Autodesk Inventor part; units mm, degrees
ref_plane "YZ Plane" through (0, 0, 0) normal (1, 0, 0) x (0, 1, 0)
ref_plane "XZ Plane" through (0, 0, 0) normal (0, 1, 0) x (-1, 0, 0)
ref_plane "XY Plane" through (0, 0, 0) normal (0, 0, 1) x (1, 0, 0)
sketch "Sketch1" plane through (0, 0, 0) normal (1, 0, 0) x (0, 1, 0)
  line L0 (-39.3892, -105) -> (-110, -20.8494)
  line L1 (-110, -20.8494) -> (-110, 0)
  line L2 (-110, 0) -> (0, 0)
  line L3 (0, 0) -> (0, -105)
  line L4 (0, -105) -> (-39.3892, -105)
  line L5 (-110, -20.8494) -> (-119.38, 0) construction
  line L6 (-119.38, 0) -> (-110, 0) construction
  line L7 (-50.8, -25.4) -> (0, -25.4) construction
  line L8 (0, -25.4) -> (0, 0) construction
  line L9 (0, 0) -> (-50.8, 0) construction
  line L10 (-50.8, 0) -> (-50.8, -25.4) construction
  line L11 (-50.8, -25.4) -> (0, 0) construction
  line L12 (0, -25.4) -> (-50.8, 0) construction
  circle A0 centre (-12.7, -12.7) radius 3
  circle A1 centre (-38.1, -12.7) radius 3
  circle A2 centre (-102.5, -49) radius 14.2875
  circle A3 centre (-25.4, -75) radius 14.2875
  circle A4 centre (-102.5, -49) radius 20
  circle A5 centre (-25.4, -75) radius 30
  line L13 (-50.8, -90.9637) -> (-50.8, -59.0363)
  line L14 (-102.5, -49) -> (-25.4, -75) construction
  point P0 (-25.4, -12.7)
  point P1 (-25.4, -25.4)
  point P2 (-103.1519, -29.0106)
  point P3 (-82.9275, -53.1131)
  point P4 (-50.8, -75)
  point P5 (-48.3813, -94.2836)
  point P6 (0, -90.9637)
  dimension "d0" = 50
  dimension "d1" = 119.38
  dimension "d2" = 50.8
  dimension "d3" = 25.4
  dimension "d4" = 25.4
  dimension "d5" = 12.7
  dimension "d6" = 6
  dimension "d7" = 6
  dimension "d8" = 28.575
  dimension "d9" = 102.5
  dimension "d10" = 49
  dimension "d13" = 110
  dimension "d16" = 60
  dimension "d17" = 25.4
  dimension "d18" = 25.4
  dimension "d20" = 40
  dimension "d44" = 81.3659
extrude "Plate1" add sketch "Sketch1" along normal blind 3.175 contours L0 A4 L1 L2 L3 A5 | A5 L13 L3 | A4 L0 A2 | L0 A2 A4 | A5 L13
fillet "Corner Round1" radius 15 4 edges at (1.5875, -82.9275, -53.1131) (1.5875, -103.1519, -29.0106) (1.5875, -110, -20.8494) (1.5875, -110, 0)
fillet "Corner Round1" radius 6 1 edges at (1.5875, 0, -90.9637)
sketch "Sketch2" plane through (0, 0, 0) normal (-1, 0, 0) x (0, 0, 1)
  circle A0 centre (-31.4501, -106.5) radius 4.5847
  circle A1 centre (-49, -102.5) radius 14.2875
  point P0 (0, 0)
  dimension "d21" = 9.1694
  dimension "d22" = 18
  dimension "d23" = 4
hole "Hole1" at (0, -106.5, -31.4501) direction (1, 0, 0) diameter 3.683 end through all
sketch "Sketch3" plane through (3.175, 0, 0) normal (1, 0, 0) x (0, 0, -1)
  circle A0 centre (75, -25.4) radius 14.2875
  circle A1 centre (75, -25.4) radius 25.4
  line L0 (49.6, -25.4) -> (100.4, -25.4)
  line L1 (92.9605, -7.4395) -> (57.0395, -7.4395)
  line L2 (75, -25.4) -> (57.0395, -7.4395)
  line L3 (92.9605, -43.3605) -> (57.0395, -43.3605)
  line L4 (75, -25.4) -> (92.9605, -43.3605)
  line L5 (25.4, -50.8) -> (0, -50.8)
  line L6 (0, -50.8) -> (0, 0)
  line L7 (0, 0) -> (25.4, 0)
  line L8 (25.4, 0) -> (25.4, -50.8)
  line L9 (25.4, -50.8) -> (0, 0) construction
  line L10 (0, -50.8) -> (25.4, 0) construction
  point P0 (12.7, -25.4)
  dimension "d31" = 50.8
  dimension "d32" = 45
  dimension "d40" = 25.4
  dimension "d41" = 50.8
hole "Hole2" at (3.175, -7.4395, -57.0395) at (3.175, -25.4, -49.6) at (3.175, -43.3605, -57.0395) at (3.175, -43.3605, -92.9605) at (3.175, -25.4, -100.4) at (3.175, -7.4395, -92.9605) direction (-1, 0, 0) diameter 5.105 end through all
equation "\"d7\" = d6"
equation "\"d29\" = Thickness"
equation "\"d14\" = Thickness"
equation "\"BendRadius\" = Thickness"
equation "\"BendReliefWidth\" = Thickness"
equation "\"BendReliefDepth\" = 0.5 * Thickness"
equation "\"CornerReliefSize\" = 4 * Thickness"
equation "\"MinimumRemnant\" = 2 * Thickness"
equation "\"TransitionRadius\" = BendRadius"
equation "\"JacobiRadiusSize\" = BendRadius"
equation "\"GapSize\" = Thickness"
properties part number "INSIDE_INTAKE_PLATE" material "Aluminum, 6061-T6"
Part model, mm, in its own coordinate system. A direction names the side the tool comes from. Round coordinates to 2 decimals unless told otherwise and drop trailing zeros. Write each loop counter-clockwise with the first axis right and the second up, starting at its lowest first coordinate (ties: lowest second). Pieces come first, ordered by that corner, then holes. Notation, with made-up numbers: (27, 19.25) -> (58, 19.25) arc R24 ccw to (58, 31.25) -> close; hole circle Ø2 at (59, -6). An arc over 180 degrees is marked (long way). Return JSON: item names as keys, results as strings. Group by question number.
Q1. Saw through at B-B on z = -49. Write the cut outline in (x, y) (1 decimal).
Q2. Probe L1, parallel to Z at x = 1.75, y = -25.4; L2, parallel to Y at x = 2.4, z = -49.6; L3, parallel to Y at x = 2.3, z = -12. List the from-to ranges inside material, lowest first. Write a range as [from, to].
Q3. Saw through at D-D on y = -102.5. Write the cut outline in (x, z) (1 decimal).
Q4. Pin check, flat tip, straight feed: pin 1 (1 mm diameter, centred on x = 1, z = -16.5, fed in from -Y). Stop position of the tip, or through.
Q5. Mould opens along Z. For faces 1 (the flat face through (2, -48, 0)), 2 (the cylindrical face through (1.565, -27.26, -89.166)), 3 (the flat face through (3.175, -48, -40)) say: pulls with the +Z half, pulls with the -Z half, needs draft (parallel to the pull), parting line crosses it, or undercut.
Q6. Saw through at C-C on x = 1.4. State how many separate pieces and enclosed holes the cut face has, plus the area to 3 significant figures.
Q7. Saw through at A-A on y = -25.4. Write the cut outline in (x, z) (1 decimal).
Q8. Which spindle directions (+Z, -Z, +X, -X, +Y, -Y) get a long thin tool onto all of the face, cutting with end or side? Do faces 4 (the cylindrical face through (1.61, -104.702, -31.849)), 5 (the flat face through (2, -110, -18)). Say none if no direction does.
Answer:
{
 "1": {"outline": "(0, -122.5) -> (3.2, -122.5) -> (3.2, -116.8) -> (0, -116.8) -> close; (0, -88.2) -> (3.2, -88.2) -> (3.2, -27.9) -> (0, -27.9) -> close; (0, -22.9) -> (3.2, -22.9) -> (3.2, 0) -> (0, 0) -> close"},
 "2": {"L1": "[-105, -102.95], [-97.85, -89.29], [-60.71, -52.15], [-47.05, 0]", "L2": "[-122.49, -116.77], [-88.23, -27.95], [-22.85, 0]", "L3": "[-109.7, -41.02], [-35.18, -15.62], [-9.78, 0]"},
 "3": {"outline": "(0, -69) -> (3.2, -69) -> (3.2, -63.3) -> (0, -63.3) -> close; (0, -34.7) -> (3.2, -34.7) -> (3.2, -2) -> (0, -2) -> close"},
 "4": {"pin 1": "y = -110"},
 "5": {"face 1": "pulls with the +Z half", "face 2": "undercut", "face 3": "needs draft"},
 "6": {"separate pieces": "1", "enclosed holes": "11", "area": "8,120 mm2"},
 "7": {"outline": "(0, -105) -> (3.2, -105) -> (3.2, -103) -> (0, -103) -> close; (0, -97.8) -> (3.2, -97.8) -> (3.2, -89.3) -> (0, -89.3) -> close; (0, -60.7) -> (3.2, -60.7) -> (3.2, -52.2) -> (0, -52.2) -> close; (0, -47) -> (3.2, -47) -> (3.2, 0) -> (0, 0) -> close"},
 "8": {"face 4": "+X, -X", "face 5": "+Z, +X, -X, -Y"}
}
